Verification items for the finished model (mm, model axes). Coordinates: 2 decimals unless noted, no trailing zeros. Use one line per item in the form item = value. Start each with the question number.
(1) Mould release check, pull along X, two halves, no side actions. Record for faces 1 (the cylindrical face through (0.806, -68.735, 2.958)), 2 (the flat face through (15, -1, 3)), 3 (the flat face through (-16, 1, 6)): released by +X, released by -X, zero draft, split by the parting line, or undercut.
(2) Material ranges on line 1 (X direction, y = -70, z = 4.25); line 2 (Y direction, x = 11, z = 3.25); line 3 (Y direction, x = -1, z = 4), recorded low to high. Write a range as [from, to].
(3) Gauge pin test, flat ends, axial feed: pin 1 Ø1.5 at (y, z) = (65, 4) entering from -X; pin 2 Ø10 at (x, y) = (-35, -65) entering from -Z; pin 3 Ø2.5 at (x, y) = (0, -70) entering from -Z. Record the tip position at first contact, or that the pin passes through.
from build123d import *

# Parameters (mm, degrees)
SKETCH1_RX          = 82.5
SKETCH1_RY          = 66.100974472
SKETCH1_R           = 1.5
BOSS_EXTRUDE1_DEPTH = 6
CUT_EXTRUDE1_DEPTH  = 10
FILLET1_R           = 5


with BuildPart() as part:
    # Sketch1 → Boss-Extrude1 (new body)
    with BuildSketch(Plane.XY):
        with Locations(Location((0, 0), (0, 0, -90))):
            Ellipse(SKETCH1_RX, SKETCH1_RY)
        with Locations((0, -70)):
            Circle(SKETCH1_R, mode=Mode.SUBTRACT)
    extrude(amount=BOSS_EXTRUDE1_DEPTH)

    # Sketch2 → Cut-Extrude1 (cut)
    with BuildSketch(Plane.XY.offset(6)):
        Polygon((15, -139.275656824), (15, 151.801672259), (87.864363855, 144.832157463), (90.234186387, -139.275656824), align=None)
    extrude(amount=-CUT_EXTRUDE1_DEPTH, mode=Mode.SUBTRACT)

    # Fillet1
    fillet1_edges = [part.edges().sort_by_distance(p)[0] for p in [
        (15, -80.347748934, 3),
        (15, 80.347748934, 3),
    ]]
    fillet(fillet1_edges, radius=FILLET1_R)


solid = part.part
Answers below:
q1.face_1 = undercut
q1.face_2 = released by +X
q1.face_3 = zero draft
q2.line_1 = [-34.98, -1.5], [1.5, 15]
q2.line_2 = [-81.35, 81.35]
q2.line_3 = [-82.49, -71.12], [-68.88, 82.49]
q3.pin_1 = -41.46
q3.pin_2 = 0
q3.pin_3 = through
